The drawing under review shows one solid part. Ordinate dimensions are in mm from its lowest x, y, z. Give positions to 0.01 mm unless a question says otherwise; leave off trailing zeros. Write each loop counter-clockwise with the first axis right and the second up, starting at its lowest first coordinate (ties: lowest second). Pieces come first, ordered by that corner, then holes. Notation, with made-up numbers: (83, 85) -> (91, 85) arc R20 cw to (91, 93) -> close; hole circle Ø4 at (26.5, 10.5). An arc over 180 degrees is marked (long way). Put each result on its own line as item: value. Start each with the question number.
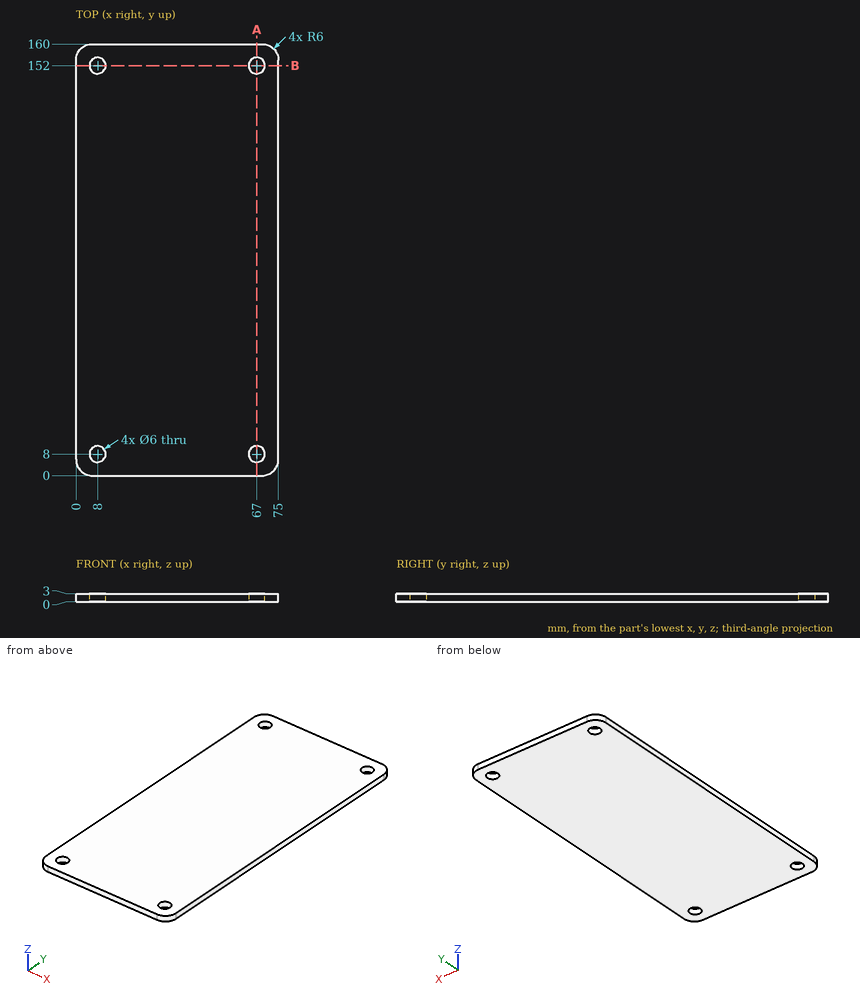
Q1. To check wall thickness, follow probe 1 along X at (y, z) = (152, 1.05); probe 2 along Y at (x, z) = (67, 2); probe 3 along Y at (x, z) = (68, 1.1). State the ranges of each line that lie inside material, in increasing order. Write a range as from..to.
Q2. For pin 1 (5 mm diameter, centred on x = 67, y = 8, fed in from +Z), flat-tipped, find the tip position at first contact; note if it passes through.
Q3. Take a section at B-B on y = 152. Give the boundary of the cut face in (x, z), then the cut area to 3 significant figures.
Q4. Take a section at A-A on x = 67. Give the boundary of the cut face in (y, z).
Result:
1. probe 1: x = 0..5, 11..64, 70..75
1. probe 2: y = 0..5, 11..149, 155..160
1. probe 3: y = 0..5.17, 10.83..149.17, 154.83..160
2. pin 1: passes through
3. outline: (0, 0) -> (5, 0) -> (5, 3) -> (0, 3) -> close; (11, 0) -> (64, 0) -> (64, 3) -> (11, 3) -> close; (70, 0) -> (75, 0) -> (75, 3) -> (70, 3) -> close
3. area: 189 mm^2
4. outline: (0, 0) -> (5, 0) -> (5, 3) -> (0, 3) -> close; (11, 0) -> (149, 0) -> (149, 3) -> (11, 3) -> close; (155, 0) -> (160, 0) -> (160, 3) -> (155, 3) -> close
